Print and shaded views of the part. All mm, measured from the part's lowest x, y and z. A direction names the side the tool comes from. Round coordinates to 2 decimals unless told otherwise and drop trailing zeros. Write each loop counter-clockwise with the first axis right and the second up, starting at its lowest first coordinate (ties: lowest second). Pieces come first, ordered by that corner, then holes. Notation, with made-up numbers: (17.25, -35.75) - (42.25, -35.75) arc R21 ccw to (42.25, -18.75) - close; hole circle Ø3 at (35.25, 46.25). An arc over 180 degrees is marked (long way). One line per item, written item: value.
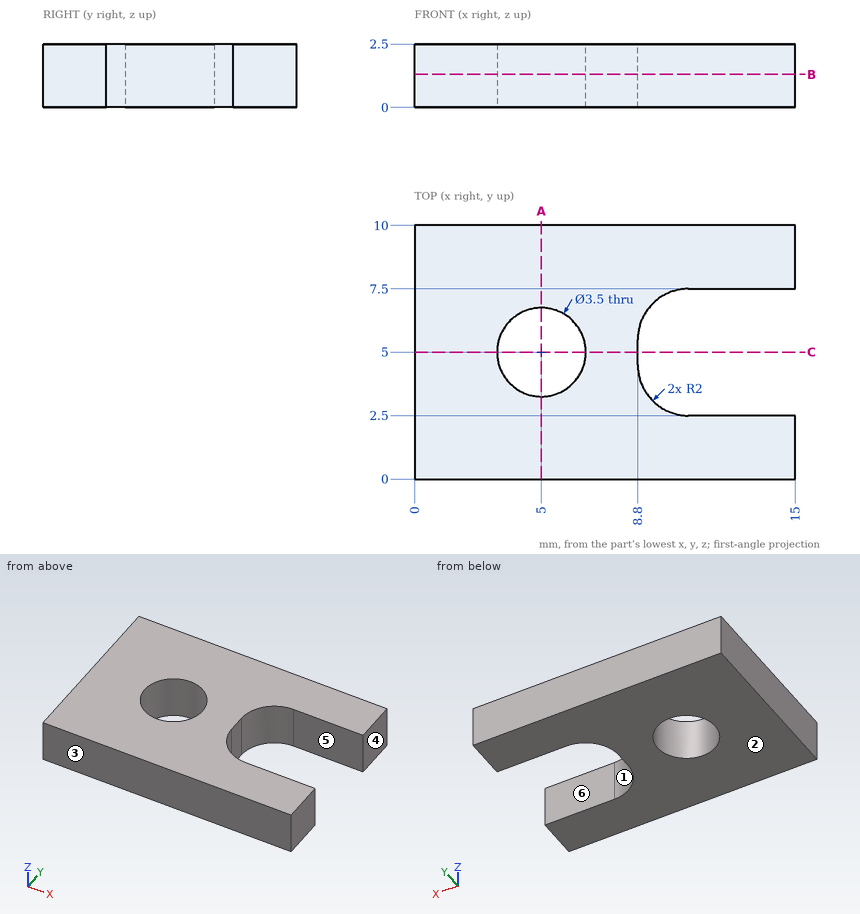
1. Band-saw the part on A-A on x = 5. Write the cut outline in (y, z), plus the area to 4 significant figures.
Report:
outline: (0, 0) - (3.25, 0) - (3.25, 2.5) - (0, 2.5) - close; (6.75, 0) - (10, 0) - (10, 2.5) - (6.75, 2.5) - close
area: 16.25 mm²
2. Band-saw the part on C-C on y = 5. Write the cut outline in (x, z).
Report:
outline: (0, 0) - (3.25, 0) - (3.25, 2.5) - (0, 2.5) - close; (6.75, 0) - (8.8, 0) - (8.8, 2.5) - (6.75, 2.5) - close
3. Band-saw the part on B-B on z = 1.3. Write the cut outline in (x, y), plus the area to 3 significant figures.
Report:
outline: (0, 0) - (15, 0) - (15, 2.5) - (10.8, 2.5) arc R2 cw to (8.8, 4.5) - (8.8, 5.5) arc R2 cw to (10.8, 7.5) - (15, 7.5) - (15, 10) - (0, 10) - close; hole circle Ø3.5 at (5, 5)
area: 111 mm²
4. Drop flat-ended pins along their axis: pin 1 (0.5 mm diameter, centred on y = 5, z = 1, fed in from +X); pin 2 (2 mm diameter, centred on x = 5, y = 5, fed in from -Z). Give the stop position or say it passes through.
Report:
pin 1: x = 8.8
pin 2: through
5. Wall check: probe 1 along Y at (x, z) = (5, 0.9); probe 2 along Y at (x, z) = (12.25, 1.5); probe 3 along X at (y, z) = (5.25, 0.85). Give the ranges that are in metal, low to high. Write a range as [from, to].
Report:
probe 1: [0, 3.25], [6.75, 10]
probe 2: [0, 2.5], [7.5, 10]
probe 3: [0, 3.27], [6.73, 8.8]
6. Mould opens along Y. For the marked faces 3, 4, 5 and 6 say: released by +Y, released by -Y, zero draft, split by the parting line, or undercut.
Report:
face 3: released by -Y
face 4: zero draft
face 5: undercut
face 6: undercut
7. Tool access for the marked faces 1 and 2: list every direction of +Z, -Z, +X, -X, +Y, -Y with a clear straight run to the whole face (end or side of a thin tool).
Report:
face 1: +Z, -Z, +X
face 2: -Z, +X, -X, +Y, -Y
